Input: part model. Units: mm. Frame: model coordinates. A direction names the side the tool comes from. Coordinates: 2 decimals unless noted, no trailing zeros. Loops run counter-clockwise (first coordinate to the right, second up) from the corner with the lowest first, then second, coordinate; pieces in that order, holes last. Notation, with made-up numbers: (19.25, -20) - (48.25, -20) arc R14 cw to (48.25, -7) - close; hole circle Ø3 at (-39, 23.25). An arc over 180 degrees is marked (long way). Use one line per item in the form item = value.
from build123d import *

# Parameters (mm, degrees)
CROQUIS1_R              = 1
CROQUIS1_W              = 10.28
CROQUIS1_H              = 2.66
SALIENTE_EXTRUIR1_DEPTH = 7.5
CROQUIS2_W              = 12.28
CROQUIS2_H              = 4.66
CORTAR_EXTRUIR1_DEPTH   = 5.5


with BuildPart() as part:
    # Croquis1 → Saliente-Extruir1 (new body)
    with BuildSketch(Plane(origin=(0, 0, 0), x_dir=(1, 0, 0), z_dir=(0, 1, 0))):
        with BuildLine():
            Line((35, -48.733971724), (30.333333333, -42.236108828))
            ThreePointArc((30.333333333, -42.236108828), (0, -52), (-30.333333333, -42.236108828))
            Line((-30.333333333, -42.236108828), (-35, -48.733971724))
            ThreePointArc((-35, -48.733971724), (0, -60), (35, -48.733971724))
        make_face()
        with Locations((-22.5, -50.18714975)):
            Circle(CROQUIS1_R, mode=Mode.SUBTRACT)
        with Locations((22.5, -50.18714975)):
            Circle(CROQUIS1_R, mode=Mode.SUBTRACT)
        with Locations((0, -55)):
            Rectangle(CROQUIS1_W, CROQUIS1_H, mode=Mode.SUBTRACT)
    extrude(amount=SALIENTE_EXTRUIR1_DEPTH)

    # Croquis2 → Cortar-Extruir1 (cut)
    with BuildSketch(Plane(origin=(0, 7.5, 0), x_dir=(1, 0, 0), z_dir=(0, 1, 0))):
        with Locations((0, -55)):
            Rectangle(CROQUIS2_W, CROQUIS2_H)
    extrude(amount=-CORTAR_EXTRUIR1_DEPTH, mode=Mode.SUBTRACT)


solid = part.part
Q1. Ray query, line 1 along Z through (x, y) = (0.5, 1.75); line 2 along Z through (x, y) = (-22.5, 3.25); line 3 along X through (y, z) = (3.5, 44.5). Return the intervals inside material, ascending. Write a range as [from, to].
Check values:
line_1 = [52, 53.67], [56.33, 60]
line_2 = [46.88, 49.19], [51.19, 55.62]
line_3 = [-31.96, -26.9], [26.9, 31.96]
Q2. Cut plane D-D, the plane y = 1. Return loops of the section in (x, z).
Check values:
outline = (-35, 48.73) - (-30.33, 42.24) arc R52 cw to (30.33, 42.24) - (35, 48.73) arc R60 ccw to start; hole circle Ø2 at (-22.5, 50.19); hole (-5.14, 53.67) - (5.14, 53.67) - (5.14, 56.33) - (-5.14, 56.33) - close; hole circle Ø2 at (22.5, 50.19)
Q3. Cut plane A-A, the plane z = 46.25. Return loops of the section in (x, y).
Check values:
outline = (-33.22, 0) - (-23.77, 0) - (-23.77, 7.5) - (-33.22, 7.5) - close; (23.77, 0) - (33.22, 0) - (33.22, 7.5) - (23.77, 7.5) - close
Q4. First-contact query: P1, Ø3.5, axis at y = 5, z = 56, coming from the +X side; P2, Ø5, axis at x = 3, z = 54, coming from the +Y side; P3, Ø2, axis at y = 0.5, z = 55.5, coming from the +X side; P4, Ø3.5, axis at y = 3.5, z = 54.5, coming from the -X side. Flat tips, straight axial feed; report the tip coordinate or a pass-through.
Check values:
P1 = 25.63
P2 = 7.5
P3 = 25.09
P4 = -28.59
Q5. Set-up query: faces 5 (the flat face through (0, 0, 53)), 6 (the flat face through (0, 1, 56.33)), 7 (the flat face through (0, 2, 57)). Return all of +Z, -Z, +X, -X, +Y, -Y with unobstructed straight access to the full face (end or side cutting, diameter ignored); none if empty.
Check values:
face_5 = +Z, -Z, +X, -X, -Y
face_6 = +Y, -Y
face_7 = +Y
Q6. Cut plane C-C, the plane y = 6.25. Return loops of the section in (x, z), then the cut area to 3 significant figures.
Check values:
outline = (-35, 48.73) - (-30.33, 42.24) arc R52 cw to (30.33, 42.24) - (35, 48.73) arc R60 ccw to start; hole circle Ø2 at (-22.5, 50.19); hole (-6.14, 52.67) - (6.14, 52.67) - (6.14, 57.33) - (-6.14, 57.33) - close; hole circle Ø2 at (22.5, 50.19)
area = 495 mm²
Q7. Pull-direction query (X, two-part tool) for faces 1 (the flat face through (32.7, 3.7, 45.53)), 2 (the flat face through (0, 5, 57.33)), 3 (the cylindrical face through (-0.523, 3.698, 59.998)), 4 (the flat face through (5.14, 1, 55)); classes: pulls with the +X half, pulls with the -X half, needs draft (parallel to the pull), parting line crosses it, or undercut.
Check values:
face_1 = pulls with the +X half
face_2 = undercut
face_3 = parting line crosses it
face_4 = undercut
Q8. Cut plane B-B, the plane x = -22.5. Return loops of the section in (y, z), then the cut area to 3 significant figures.
Check values:
outline = (0, 46.88) - (7.5, 46.88) - (7.5, 49.19) - (0, 49.19) - close; (0, 51.19) - (7.5, 51.19) - (7.5, 55.62) - (0, 55.62) - close
area = 50.6 mm²
